from build123d import *

# Parameters (mm, degrees)
BOSS_EXTRUDE1_DEPTH = 2
SKETCH2_R           = 7.999999999999998
BOSS_EXTRUDE2_DEPTH = 12
SKETCH3_R           = 6.499999999999999
SKETCH3_R_2         = 6.5
CUT_EXTRUDE1_DEPTH  = 0.5
BOSS_EXTRUDE3_DEPTH = 4
FILLET1_R           = 0.1
FILLET2_R           = 0.5


with BuildPart() as part:
    # Sketch1 → Boss-Extrude1 (new body)
    with BuildSketch(Plane.XY):
        Polygon((22.499999999999993, -10.249999999999996), (-22.500000000000007, -10.25), (-22.500000000000007, 10.25), (22.499999999999993, 10.250000000000005), align=None)
    extrude(amount=BOSS_EXTRUDE1_DEPTH)

    # Sketch2 → Boss-Extrude2 (add)
    with BuildSketch(Plane.XY.offset(2)):
        with Locations((-12.750000000000004, 1.12e-15)):
            Circle(SKETCH2_R)
        with Locations((12.749999999999998, 1.12e-15)):
            Circle(SKETCH2_R)
    extrude(amount=BOSS_EXTRUDE2_DEPTH)

    # Sketch3 → Cut-Extrude1 (cut)
    with BuildSketch(Plane.XY.offset(14)):
        with Locations((-12.750000000000004, 1.12e-15)):
            Circle(SKETCH3_R)
        with Locations(Location((12.749999999999991, -2.316e-14, 0), (0, 0, 180))):
            Circle(SKETCH3_R_2)
    extrude(amount=-CUT_EXTRUDE1_DEPTH, mode=Mode.SUBTRACT)

    # Sketch4 → Boss-Extrude3 (add)
    with BuildSketch(Plane.XY.offset(2)):
        with BuildLine():
            Line((3.5999999999999757, -10.249999999999995), (-3.5999999999999965, -10.249999999999996))
            ThreePointArc((-3.5999999999999965, -10.249999999999996), (-4.943502884254451, -9.693502884254437), (-5.50000000000001, -8.349999999999982))
            Line((-5.50000000000001, -8.349999999999982), (-5.50000000000001, -8.15000000000001))
            ThreePointArc((-5.50000000000001, -8.15000000000001), (-4.943502884254451, -6.8064971157455565), (-3.5999999999999965, -6.2499999999999964))
            Line((-3.5999999999999965, -6.2499999999999964), (3.5999999999999757, -6.249999999999996))
            ThreePointArc((3.5999999999999757, -6.249999999999996), (4.943502884254429, -6.806497115745555), (5.499999999999989, -8.150000000000007))
            Line((5.499999999999989, -8.150000000000007), (5.499999999999989, -8.349999999999982))
            ThreePointArc((5.499999999999989, -8.349999999999982), (4.943502884254429, -9.693502884254436), (3.5999999999999757, -10.249999999999995))
        make_face()
    extrude(amount=BOSS_EXTRUDE3_DEPTH)

    # Fillet1
    fillet1_edges = [part.edges().sort_by_distance(p)[0] for p in [
        (4.94350288425443, -9.693502884254436, 6),
        (5.499999999999989, -8.249999999999995, 6),
        (4.943502884254428, -6.806497115745555, 6),
        (-1.021e-14, -6.2499999999999964, 6),
        (-4.94350288425445, -6.8064971157455565, 6),
        (-5.50000000000001, -8.249999999999996, 6),
        (-4.943502884254451, -9.693502884254437, 6),
        (-1.066e-14, -10.249999999999996, 6),
    ]]
    fillet(fillet1_edges, radius=FILLET1_R)

    # Fillet2
    fillet2_edges = [part.edges().sort_by_distance(p)[0] for p in [
        (4.94350288425443, -9.693502884254436, 2),
        (5.499999999999989, -8.249999999999995, 2),
        (4.943502884254428, -6.806497115745555, 2),
        (-1.021e-14, -6.2499999999999964, 2),
        (-4.94350288425445, -6.8064971157455565, 2),
        (-5.50000000000001, -8.249999999999996, 2),
        (-4.943502884254451, -9.693502884254437, 2),
    ]]
    fillet(fillet2_edges, radius=FILLET2_R)


solid = part.part
Geometry: final body of the model. Coordinates: model frame, mm. A direction names the side the tool comes from. Round coordinates to 2 decimals unless told otherwise and drop trailing zeros. Order: outer loops, then holes, each group sorted by start corner. A loop starts at its lowest first (then second) coordinate and runs counter-clockwise, first axis right, second up. Notation, with made-up numbers: (71.5, 65) - (126.5, 65) arc R15 ccw to (126.5, 93) - close; hole circle Ø11 at (38, 45.25). An arc over 180 degrees is marked (long way). Write each question's results on one line, items separated by ' | '.
Item 1: First-contact query: pin 1 Ø5 at (x, z) = (5, 11) entering from -Y; pin 2 Ø10.5 at (x, y) = (-12.75, 0) entering from +Z; pin 3 Ø1.9 at (x, y) = (-2, -7.5) entering from +Z. Flat tips, straight axial feed; report the tip coordinate or a pass-through.
Completed:
pin 1: y = -6.04 | pin 2: z = 13.5 | pin 3: z = 6
Item 2: Section A-A, the plane y = 0. Return the cut outline in (x, z).
Completed:
outline: (-22.5, 0) - (22.5, 0) - (22.5, 2) - (20.75, 2) - (20.75, 14) - (19.25, 14) - (19.25, 13.5) - (6.25, 13.5) - (6.25, 14) - (4.75, 14) - (4.75, 2) - (-4.75, 2) - (-4.75, 14) - (-6.25, 14) - (-6.25, 13.5) - (-19.25, 13.5) - (-19.25, 14) - (-20.75, 14) - (-20.75, 2) - (-22.5, 2) - close
Item 3: Reachability of faces 4 (the flat face through (0, -6.25, 4)), 5 (the cylindrical face through (-19.244, 0.286, 13.754)), 6 (the cylindrical face through (4.958, -9.679, 4.176)), 7 (the flat face through (0, 10.25, 1)), 8 (the cylindrical face through (-4.929, -9.708, 4.176)) from +Z, -Z, +X, -X, +Y, -Y: full face, straight path, thin tool, end or side. Return the list, or none.
Completed:
face 4: +Z, +Y | face 5: +Z | face 6: +Z, +X, -Y | face 7: +Z, -Z, +X, -X, +Y | face 8: +Z, -X, -Y
Item 4: Mould query, pull axis X, two halves, no side actions, for faces 1 (the flat face through (22.5, 0, 1)), 2 (the flat face through (13, 0, 13.5)), 3 (the flat face through (-13, 7, 14)). Classes: pulls with the +X half, pulls with the -X half, needs draft (parallel to the pull), parting line crosses it, or undercut.
Completed:
face 1: pulls with the +X half | face 2: undercut | face 3: needs draft
Item 5: Section D-D, the plane x = -8. Return the cut outline in (y, z).
Completed:
outline: (-10.25, 0) - (10.25, 0) - (10.25, 2) - (6.44, 2) - (6.44, 14) - (4.44, 14) - (4.44, 13.5) - (-4.44, 13.5) - (-4.44, 14) - (-6.44, 14) - (-6.44, 2) - (-10.25, 2) - close
Item 6: Material intervals for line 1 along Y through (x, z) = (12.75, 13.7); line 2 along X through (y, z) = (-7, 5.5); line 3 along Z through (x, y) = (-8, -1.5), sorted ascending. Write a range as [from, to].
Completed:
line 1: [-8, -6.5], [6.5, 8] | line 2: [-16.62, -8.88], [-5.11, 5.11], [8.88, 16.62] | line 3: [0, 13.5]
Item 7: Section C-C, the plane x = -12.75. Return the cut outline in (y, z).
Completed:
outline: (-10.25, 0) - (10.25, 0) - (10.25, 2) - (8, 2) - (8, 14) - (6.5, 14) - (6.5, 13.5) - (-6.5, 13.5) - (-6.5, 14) - (-8, 14) - (-8, 2) - (-10.25, 2) - close
Item 8: Section B-B, the plane z = 12.25. Return the cut outline in (x, y), and give its area (3 significant figures).
Completed:
outline: circle Ø16 at (-12.75, 0); circle Ø16 at (12.75, 0) | area: 402 mm^2
